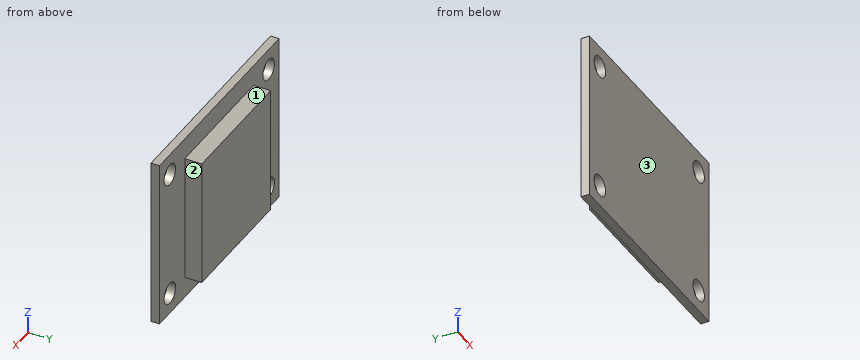
from build123d import *

# Parameters (mm, degrees)
SKETCH1_W           = 26
SKETCH1_H           = 20
BOSS_EXTRUDE1_DEPTH = 1
SKETCH2_R           = 1.25
CUT_EXTRUDE1_DEPTH  = 1
SKETCH3_W           = 15
SKETCH3_H           = 15
BOSS_EXTRUDE2_DEPTH = 3


with BuildPart() as part:
    # Sketch1 → Boss-Extrude1 (new body)
    with BuildSketch(Plane(origin=(0, 0, 0), x_dir=(1, 0, 0), z_dir=(0, 1, 0))):
        Rectangle(SKETCH1_W, SKETCH1_H)
    extrude(amount=BOSS_EXTRUDE1_DEPTH)

    # Sketch2 → Cut-Extrude1 (cut)
    with BuildSketch(Plane(origin=(0, 0, 0), x_dir=(1, 0, 0), z_dir=(0, 1, 0))):
        with Locations((-10.75, 7.5)):
            Circle(SKETCH2_R)
        with Locations((-10.75, -7.5)):
            Circle(SKETCH2_R)
        with Locations((10.75, -7.5)):
            Circle(SKETCH2_R)
        with Locations((10.75, 7.5)):
            Circle(SKETCH2_R)
    extrude(amount=CUT_EXTRUDE1_DEPTH, mode=Mode.SUBTRACT)

    # Sketch3 → Boss-Extrude2 (add)
    with BuildSketch(Plane(origin=(0, 0, 0), x_dir=(1, 0, 0), z_dir=(0, 1, 0))):
        Rectangle(SKETCH3_W, SKETCH3_H)
    extrude(amount=BOSS_EXTRUDE2_DEPTH)


solid = part.part
Geometry: final body of the model. Coordinates: model frame, mm. Face numbers are marked on the shaded views. A direction names the side the tool comes from. Round coordinates to 2 decimals unless told otherwise and drop trailing zeros. Loops run counter-clockwise (first coordinate to the right, second up) from the corner with the lowest first, then second, coordinate; pieces in that order, holes last. Notation, with made-up numbers: (-36.5, -21) -> (4.5, -21) arc R8 ccw to (4.5, -9) -> close; hole circle Ø1 at (-2.75, 35.25). An arc over 180 degrees is marked (long way). One line per question, with ' | ' between items. Start each with the question number.
1. Line query: line 1 along Z through (x, y) = (10.75, 0.5); line 2 along X through (y, z) = (0.65, -7.5); line 3 along Z through (x, y) = (-2.75, 1.05). Output: solid intervals per line, ascending. Write a range as [from, to].
2. Set-up query: the marked faces 1, 2 and 3. Return all of +Z, -Z, +X, -X, +Y, -Y with unobstructed straight access to the full face (end or side cutting, diameter ignored); none if empty.
3. Section C-C on x = 4.25. Output: boundary loops of the cut face in (y, z).
4. Section A-A on x = 10.75. Output: boundary loops of the cut face in (y, z).
5. Section D-D on z = -3.75. Output: boundary loops of the cut face in (x, y), and give its area (3 significant figures).
6. Contact query for flat-ended pins moving along their axis: pin 1 (0.6 mm diameter, centred on y = 2, z = -2.5, fed in from +X); pin 2 (3 mm diameter, centred on x = -10.75, z = -7.5, fed in from +Y); pin 3 (0.6 mm diameter, centred on x = -1.5, y = 2.5, fed in from -Z); pin 4 (2 mm diameter, centred on x = 10.75, z = 7.5, fed in from -Y). Output: stop coordinate, or through.
7. Section B-B on y = 0.35. Output: boundary loops of the cut face in (x, z).
Returned:
1) line 1: z = [-10, -8.75], [-6.25, 6.25], [8.75, 10] | line 2: x = [-13, -12], [-9.5, 9.5], [12, 13] | line 3: z = [-7.5, 7.5]
2) face 1: +Z, +X, -X, +Y | face 2: +Z, -Z, +X, +Y | face 3: +Z, -Z, +X, -X, -Y
3) outline: (0, -10) -> (1, -10) -> (1, -7.5) -> (3, -7.5) -> (3, 7.5) -> (1, 7.5) -> (1, 10) -> (0, 10) -> close
4) outline: (0, -10) -> (1, -10) -> (1, -8.75) -> (0, -8.75) -> close; (0, -6.25) -> (1, -6.25) -> (1, 6.25) -> (0, 6.25) -> close; (0, 8.75) -> (1, 8.75) -> (1, 10) -> (0, 10) -> close
5) outline: (-13, 0) -> (13, 0) -> (13, 1) -> (7.5, 1) -> (7.5, 3) -> (-7.5, 3) -> (-7.5, 1) -> (-13, 1) -> close | area: 56.0 mm2
6) pin 1: stops at x = 7.5 | pin 2: stops at y = 1 | pin 3: stops at z = -7.5 | pin 4: passes through
7) outline: (-13, -10) -> (13, -10) -> (13, 10) -> (-13, 10) -> close; hole circle Ø2.5 at (-10.75, -7.5); hole circle Ø2.5 at (-10.75, 7.5); hole circle Ø2.5 at (10.75, -7.5); hole circle Ø2.5 at (10.75, 7.5)
